The model under review builds one solid part; all positions refer to its coordinate system, in mm. Round coordinates to 2 decimals unless told otherwise and drop trailing zeros. Order: outer loops, then holes, each group sorted by start corner. A loop starts at its lowest first (then second) coordinate and runs counter-clockwise, first axis right, second up. Notation, with made-up numbers: M 19,-12.75 L 50,-12.75 A12 cw 50,-3.75 Z; hole C 46.5,-36.5 d3. An arc over 180 degrees is marked long. Use a Markdown table: item, result. Add a question column.
1. Insertion check: P1, Ø1, axis at x = -1.5, z = 33, coming from the -Y side; P2, Ø1.5, axis at x = 1.5, z = 40.5, coming from the -Y side; P3, Ø1.5, axis at y = -1, z = 35, coming from the -X side. Each pin has a flat end and moves straight along its axis. Give the tip position at first contact, or say it passes through.
2. Consider section D-D on z = 42. State the section outline as (x, y) points, then the cut area to 3 significant figures.
3. Consider section A-A on x = 0.5. Count the separate pieces of the cut face and the enclosed holes in it, then the cut area to 3 significant figures.
4. To check wall thickness, follow probe 1 along Z at (x, y) = (-1, -1); probe 2 along Y at (x, z) = (0, 49.75); probe 3 along Z at (x, y) = (0, -0.5). State the ranges of each line that lie inside material, in increasing order.
5. Consider section B-B on z = 4. State the section outline as (x, y) points, then the cut area to 3 significant figures.
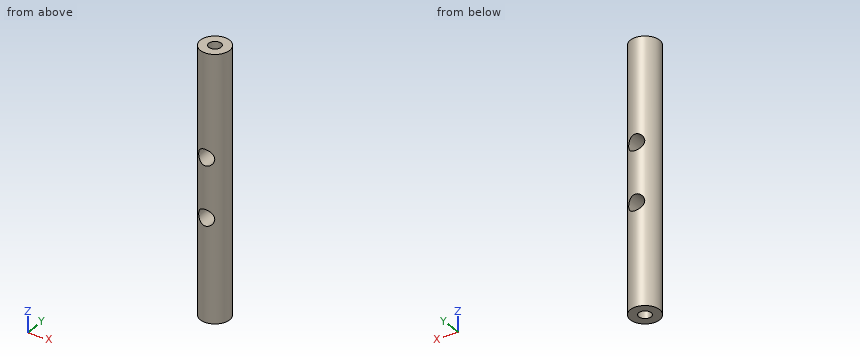
from build123d import *

# Parameters (mm, degrees)
SKETCH_1_R      = 3
EXTRUDE_1_DEPTH = 53.8
M4X0_7_1_D      = 3.3
M4X0_7_1_DEPTH  = 11.5
M4X0_7_1_TIP    = 0.991420021
M3X0_5_2_D      = 2.5
M3X0_5_2_DEPTH  = 8.5
M3X0_5_2_TIP    = 0.751075774


with BuildPart() as part:
    # ｽｹｯﾁ1 → ﾎﾞｽ - 押し出し1 (new body)
    with BuildSketch(Plane.XY):
        Circle(SKETCH_1_R)
    extrude(amount=EXTRUDE_1_DEPTH)

    # M4x0.7 ねじ穴1
    with Locations(Plane(origin=(0.029051092, 2.999859336, 32.9), x_dir=(0.999953112, -0.009683697, 0), z_dir=(0.009683697, 0.999953112, 0))):
        with Locations((0, 0), (0, 12)):
            Hole(M4X0_7_1_D / 2, depth=M4X0_7_1_DEPTH)
            with Locations((0, 0, -(M4X0_7_1_DEPTH + M4X0_7_1_TIP / 2))):  # 118° drill point
                Cone(0, M4X0_7_1_D / 2, M4X0_7_1_TIP, mode=Mode.SUBTRACT)

    # ｽｹｯﾁ7 → M3x0.5 ねじ穴1 (revolve, cut)
    with BuildSketch(Plane(origin=(0, 0, 53.8), x_dir=(0, -1, 0), z_dir=(1, 0, 0))):
        Polygon((0, 0), (0, 9.251075774), (1.25, 8.5), (1.25, 0), align=None)
    revolve(axis=Axis((0, 0, 60.15), (0, 0, -1)), mode=Mode.SUBTRACT)

    # M3x0.5 ねじ穴2
    with Locations(Plane(origin=(0, 0, 0), x_dir=(-1, 0, 0), z_dir=(0, 0, -1))):
        with Locations((0, 0)):
            Hole(M3X0_5_2_D / 2, depth=M3X0_5_2_DEPTH)
            with Locations((0, 0, -(M3X0_5_2_DEPTH + M3X0_5_2_TIP / 2))):  # 118° drill point
                Cone(0, M3X0_5_2_D / 2, M3X0_5_2_TIP, mode=Mode.SUBTRACT)


solid = part.part
Answer block:
| question | item | result |
|---|---|---|
| 1 | P1 | y = -2.56 |
| 1 | P2 | y = -2.9 |
| 1 | P3 | x = -2.99 |
| 2 | outline | C 0,0 d6 |
| 2 | area | 28.3 mm^2 |
| 3 | separate pieces | 3 |
| 3 | enclosed holes | 0 |
| 3 | area | 241 mm^2 |
| 4 | probe 1 | 0 to 19.58, 22.22 to 31.58, 34.22 to 53.8 |
| 4 | probe 2 | -3 to -1.25, 1.25 to 3 |
| 4 | probe 3 | 8.95 to 19.25, 22.55 to 31.25, 34.55 to 44.85 |
| 5 | outline | C 0,0 d6; hole C 0,0 d2.5 |
| 5 | area | 23.4 mm^2 |
